Work out the finished part from the listing and answer in its coordinate system (mm). Face numbers are marked on the shaded views. A direction names the side the tool comes from. Coordinates: 2 decimals unless noted, no trailing zeros. Loops run counter-clockwise (first coordinate to the right, second up) from the corner with the lowest first, then second, coordinate; pieces in that order, holes last. Notation, with made-up numbers: (21, 20) - (30, 20) arc R31 cw to (30, 51) - close; hole circle Ø7 at (-28, 26.5). An arc over 180 degrees is marked (long way). Write each question's results on one line, items separated by ' | '. Start each with the question number.
1. Which of the six approach directions +Z, -Z, +X, -X, +Y, -Y give full straight-line access (tool end or side, diameter ignored) to the marked faces 4, 5 and 6?
2. A cutting plane is placed at C-C on x = -4.5. Determine the outline of the cut face in (y, z) (1 decimal), then the cut area to 3 significant figures.
3. Determine the mould class of the marked faces 1, 2 and 3 for opening direction Z: released by +Z, released by -Z, zero draft, split by the parting line, or undercut.
4. Find the intervals of material crossed by line 1 along Z through (x, y) = (17.5, 253.5) (3 decimals); line 2 along X through (y, z) = (226, 249.5); line 3 along X through (y, z) = (230, 40.5), in increasing order. Write a range as [from, to].
5. Each of these flat-tipped pins is pushed along its axis until it touches: P1, Ø3, axis at x = 28.5, y = 254.5, coming from the +Z side (3 decimals); P2, Ø12, axis at y = 229, z = 60.5, coming from the -X side; P3, Ø10, axis at y = 257.5, z = 184.5, coming from the +X side; P4, Ø8, axis at x = -18.5, z = 131.5, coming from the +Y side. Where does it stop, or does it pass through?
6. A cutting plane is placed at B-B on y = 266. Determine the outline of the cut face in (x, z) (3 decimals), then the cut area to 3 significant figures.
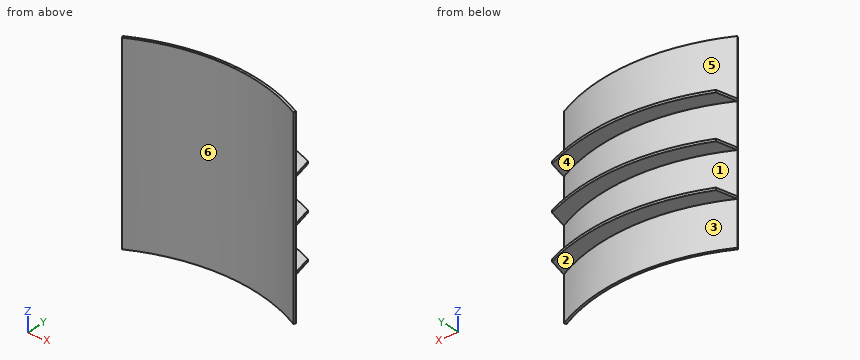
from build123d import *

# Parameters (mm, degrees)
BOSS_EXTRUDE1_DEPTH = 260
BOSS_EXTRUDE2_START = 60
BOSS_EXTRUDE2_DEPTH = 3.175
LPATTERN1_COUNT     = 3
LPATTERN1_PITCH     = 60


with BuildPart() as part:
    # Sketch1 → Boss-Extrude1 (new body)
    with BuildSketch(Plane.XY):
        with BuildLine():
            Line((-116.4605, 224.79887136), (-115, 221.979728804))
            ThreePointArc((-115, 221.979728804), (0, 250), (115, 221.979728804))
            Line((115, 221.979728804), (116.4605, 224.79887136))
            ThreePointArc((116.4605, 224.79887136), (0, 253.175), (-116.4605, 224.79887136))
        make_face()
    extrude(amount=BOSS_EXTRUDE1_DEPTH)

    # Sketch2 → Boss-Extrude2 (add)
    with BuildSketch(Plane.XY.offset(BOSS_EXTRUDE2_START)):
        with BuildLine():
            Line((-110, 252.041663223), (-116.4605, 224.79887136))
            ThreePointArc((-116.4605, 224.79887136), (0, 253.175), (116.4605, 224.79887136))
            Line((116.4605, 224.79887136), (110, 252.041663223))
            ThreePointArc((110, 252.041663223), (0, 275), (-110, 252.041663223))
        make_face()
    boss_extrude2 = extrude(amount=BOSS_EXTRUDE2_DEPTH)

    # LPattern1: Boss-Extrude2 ×3
    with Locations(*[(0, 0, i * LPATTERN1_PITCH) for i in range(1, LPATTERN1_COUNT)]):
        add(boss_extrude2)


solid = part.part
Values:
1) face 4: +Y | face 5: +Z, +Y | face 6: +Z, -Z, -Y
2) outline: (250, 0) - (253.1, 0) - (253.1, 60) - (275, 60) - (275, 63.2) - (253.1, 63.2) - (253.1, 120) - (275, 120) - (275, 123.2) - (253.1, 123.2) - (253.1, 180) - (275, 180) - (275, 183.2) - (253.1, 183.2) - (253.1, 260) - (250, 260) - close | area: 1,030 mm^2
3) face 1: undercut | face 2: released by -Z | face 3: zero draft
4) line 1: [60, 63.175], [120, 123.175], [180, 183.175] | line 2: [-114.11, -106.88], [106.88, 114.11] | line 3: [-105.82, -97.98], [97.98, 105.82]
5) P1: z = 183.175 | P2: x = -116.46 | P3: x = 108.53 | P4: y = 252.76
6) outline: (-69.778, 60) - (69.778, 60) - (69.778, 63.175) - (-69.778, 63.175) - close; (-69.778, 120) - (69.778, 120) - (69.778, 123.175) - (-69.778, 123.175) - close; (-69.778, 180) - (69.778, 180) - (69.778, 183.175) - (-69.778, 183.175) - close | area: 1,330 mm^2
